from build123d import *

# Parameters (mm, degrees)
F0_W     = 25
F0_H     = 25
F0_R     = 1.6
F0_R_2   = 7
F1_DEPTH = 2
F2_R     = 9
F2_R_2   = 7
F3_DEPTH = 9


with BuildPart() as f1:
    # F0 (on Top) → F1 (new body)
    with BuildSketch(Plane.XY):
        Rectangle(F0_W, F0_H)
        with Locations((-8.838835, -8.838835)):
            Circle(F0_R, mode=Mode.SUBTRACT)
        Circle(F0_R_2, mode=Mode.SUBTRACT)
        with Locations((8.838835, 8.838835)):
            Circle(F0_R, mode=Mode.SUBTRACT)
    extrude(amount=F1_DEPTH)

    # F2 (on face) → F3 (join)
    with BuildSketch(Plane.XY.offset(2)):
        Circle(F2_R)
        Circle(F2_R_2, mode=Mode.SUBTRACT)
    extrude(amount=F3_DEPTH)


solid = f1.part
Geometry check sheet. Reference: the model listing, model coordinates, mm. A direction names the side the tool comes from. Give positions to 0.01 mm unless a question says otherwise; leave off trailing zeros. Order: outer loops, then holes, each group sorted by start corner. A loop starts at its lowest first (then second) coordinate and runs counter-clockwise, first axis right, second up. Notation, with made-up numbers: M -10.75,-10.75 L -6.75,-10.75 A28 cw -6.75,21.25 Z; hole C -18,11 d3. An arc over 180 degrees is marked long. Use a Markdown table: item, result.
Item 1: Material ranges on line 1 along Y through (x, z) = (-8.75, 0.75); line 2 along Y through (x, z) = (0, 4.5); line 3 along Z through (x, y) = (-11, 3), recorded low to high.
Answers follow:
| item | result |
|---|---|
| line 1 | y = -12.5 to -10.44, -7.24 to 12.5 |
| line 2 | y = -9 to -7, 7 to 9 |
| line 3 | z = 0 to 2 |
Item 2: Draft check along X on faces 3 (the flat face through (0, -7.3, 11)), 4 (the cylindrical face through (6.466, -2.681, 5.423)), 5 (the cylindrical face through (8.631, 10.425, 0.986)), 6 (the flat face through (-12.5, 0, 1)). Enter one of: +X half, -X half, draft (parallel to the pull), parting line (faces both ways), or undercut.
Answers follow:
| item | result |
|---|---|
| face 3 | draft |
| face 4 | undercut |
| face 5 | undercut |
| face 6 | -X half |
Item 3: Tool access check on faces 1 (the cylindrical face through (-10.437, -8.768, 0.986)), 2 (the flat face through (-9, 3, 2)). Record the directions out of +Z, -Z, +X, -X, +Y, -Y that give a thin tool (end or side, any length) a straight path to the whole face; none if there is none.
Answers follow:
| item | result |
|---|---|
| face 1 | +Z, -Z |
| face 2 | +Z |
Item 4: Section check C-C (z = 1). Record the cut outline in (x, y), and give its area (3 significant figures).
Answers follow:
| item | result |
|---|---|
| outline | M -12.5,-12.5 L 12.5,-12.5 L 12.5,12.5 L -12.5,12.5 Z; hole C -8.84,-8.84 d3.2; hole C 0,0 d14; hole C 8.84,8.84 d3.2 |
| area | 455 mm2 |
Item 5: Section check A-A (x = 0). Record the cut outline in (y, z).
Answers follow:
| item | result |
|---|---|
| outline | M -12.5,0 L -7,0 L -7,11 L -9,11 L -9,2 L -12.5,2 Z; M 7,0 L 12.5,0 L 12.5,2 L 9,2 L 9,11 L 7,11 Z |
Item 6: Section check D-D (z = 5.5). Record the cut outline in (x, y).
Answers follow:
| item | result |
|---|---|
| outline | C 0,0 d18; hole C 0,0 d14 |
Item 7: Depth check by flat-ended pin: P1, Ø4, axis at y = 0, z = 4.5, coming from the -X side; P2, Ø3, axis at y = -3.5, z = 4.5, coming from the +X side; P3, Ø1, axis at x = -1, y = 4.5, coming from the +Z side; P4, Ø6, axis at x = 7.5, z = 5.5, coming from the +Y side. Enter the tip coordinate at first touch or a pass-through.
Answers follow:
| item | result |
|---|---|
| P1 | stops at x = -9 |
| P2 | stops at x = 8.77 |
| P3 | passes through |
| P4 | stops at y = 7.79 |
